from build123d import *

# Parameters (mm, degrees)
SKETCH1_W               = 500
SKETCH1_H               = 200
BOSS_EXTRUDE1_DEPTH     = 100
SKETCH2_R               = 40
BOSS_EXTRUDE2_DEPTH     = 10
SKETCH5_R               = 1.5
CUT_EXTRUDE3_DEPTH      = 20
CIRPATTERN2_COUNT       = 3
MIRROR4_COPY_1_SKETCH_R = 1.5
MIRROR4_COPY_1_DEPTH    = 20
MIRROR4_COPY_2_SKETCH_R = 1.5
MIRROR4_COPY_2_DEPTH    = 20
MIRROR5_COPY_1_SKETCH_R = 1.5
MIRROR5_COPY_1_DEPTH    = 20
MIRROR5_COPY_2_SKETCH_R = 1.5
MIRROR5_COPY_2_DEPTH    = 20
MIRROR5_COPY_3_SKETCH_R = 40
MIRROR5_COPY_3_DEPTH    = 10
MIRROR5_COPY_4_SKETCH_R = 1.5
MIRROR5_COPY_4_DEPTH    = 20
MIRROR5_COPY_5_SKETCH_R = 1.5
MIRROR5_COPY_5_DEPTH    = 20
MIRROR5_COPY_6_SKETCH_R = 1.5
MIRROR5_COPY_6_DEPTH    = 20


with BuildPart() as part:
    # Sketch1 → Boss-Extrude1 (new body)
    with BuildSketch(Plane(origin=(0, 0, 0), x_dir=(1, 0, 0), z_dir=(0, 1, 0))):
        Rectangle(SKETCH1_W, SKETCH1_H)
    extrude(amount=BOSS_EXTRUDE1_DEPTH)

    # Sketch2 → Boss-Extrude2 (add)
    with BuildSketch(Plane.XY.offset(100)):
        with Locations(Location((-170, 50, 0), (0, 0, 180))):
            Circle(SKETCH2_R)
    boss_extrude2 = extrude(amount=BOSS_EXTRUDE2_DEPTH)

    # Sketch5 → Cut-Extrude3 (cut)
    with BuildSketch(Plane.XY.offset(110)):
        with Locations((-170, 86)):
            Circle(SKETCH5_R)
    cut_extrude3 = extrude(amount=-CUT_EXTRUDE3_DEPTH, mode=Mode.SUBTRACT)

    # CirPattern2: Cut-Extrude3 ×3 about axis
    cirpattern2_axis = Axis((-170, 50, 0), (0, 0, 1))
    for i in range(1, CIRPATTERN2_COUNT):
        add(cut_extrude3.rotate(cirpattern2_axis, i * 360 / CIRPATTERN2_COUNT), mode=Mode.SUBTRACT)

    # Mirror4: Boss-Extrude2, Cut-Extrude3 across plane
    add(boss_extrude2.mirror(Plane(origin=(0, 0, 0), x_dir=(0, 0, 1), z_dir=(1, 0, 0))))
    add(cut_extrude3.mirror(Plane(origin=(0, 0, 0), x_dir=(0, 0, 1), z_dir=(1, 0, 0))), mode=Mode.SUBTRACT)

    # Mirror4 copy 1 sketch → Mirror4 copy 1 (cut)
    with BuildSketch(Plane(origin=(211.698729811, 222.224318643, 110), x_dir=(0.4999999999999998, 0.8660254037844387, 0), z_dir=(0, 0, 1))):
        with Locations((-170, -86)):
            Circle(MIRROR4_COPY_1_SKETCH_R)
    extrude(amount=-MIRROR4_COPY_1_DEPTH, mode=Mode.SUBTRACT)

    # Mirror4 copy 2 sketch → Mirror4 copy 2 (cut)
    with BuildSketch(Plane(origin=(298.301270189, -72.224318643, 110), x_dir=(0.5000000000000004, -0.8660254037844384, 0), z_dir=(0, 0, 1))):
        with Locations((-170, -86)):
            Circle(MIRROR4_COPY_2_SKETCH_R)
    extrude(amount=-MIRROR4_COPY_2_DEPTH, mode=Mode.SUBTRACT)

    # Mirror5: Boss-Extrude2, Cut-Extrude3 across plane
    add(boss_extrude2.mirror(Plane.XY))
    add(cut_extrude3.mirror(Plane.XY), mode=Mode.SUBTRACT)

    # Mirror5 copy 1 sketch → Mirror5 copy 1 (cut)
    with BuildSketch(Plane(origin=(-211.698729811, 222.224318643, -110), x_dir=(-0.4999999999999998, 0.8660254037844387, 0), z_dir=(0, 0, -1))):
        with Locations((-170, -86)):
            Circle(MIRROR5_COPY_1_SKETCH_R)
    extrude(amount=-MIRROR5_COPY_1_DEPTH, mode=Mode.SUBTRACT)

    # Mirror5 copy 2 sketch → Mirror5 copy 2 (cut)
    with BuildSketch(Plane(origin=(-298.301270189, -72.224318643, -110), x_dir=(-0.5000000000000004, -0.8660254037844384, 0), z_dir=(0, 0, -1))):
        with Locations((-170, -86)):
            Circle(MIRROR5_COPY_2_SKETCH_R)
    extrude(amount=-MIRROR5_COPY_2_DEPTH, mode=Mode.SUBTRACT)

    # Mirror5 copy 3 sketch → Mirror5 copy 3 (add)
    with BuildSketch(Plane(origin=(0, 0, -100), x_dir=(-1, 0, 0), z_dir=(0, 0, -1))):
        with Locations(Location((-170, 50, 0), (0, 0, 180))):
            Circle(MIRROR5_COPY_3_SKETCH_R)
    extrude(amount=MIRROR5_COPY_3_DEPTH)

    # Mirror5 copy 4 sketch → Mirror5 copy 4 (cut)
    with BuildSketch(Plane(origin=(0, 0, -110), x_dir=(-1, 0, 0), z_dir=(0, 0, -1))):
        with Locations((-170, 86)):
            Circle(MIRROR5_COPY_4_SKETCH_R)
    extrude(amount=-MIRROR5_COPY_4_DEPTH, mode=Mode.SUBTRACT)

    # Mirror5 copy 5 sketch → Mirror5 copy 5 (cut)
    with BuildSketch(Plane(origin=(211.698729811, 222.224318643, -110), x_dir=(0.4999999999999998, 0.8660254037844387, 0), z_dir=(0, 0, -1))):
        with Locations((-170, 86)):
            Circle(MIRROR5_COPY_5_SKETCH_R)
    extrude(amount=-MIRROR5_COPY_5_DEPTH, mode=Mode.SUBTRACT)

    # Mirror5 copy 6 sketch → Mirror5 copy 6 (cut)
    with BuildSketch(Plane(origin=(298.301270189, -72.224318643, -110), x_dir=(0.5000000000000004, -0.8660254037844384, 0), z_dir=(0, 0, -1))):
        with Locations((-170, 86)):
            Circle(MIRROR5_COPY_6_SKETCH_R)
    extrude(amount=-MIRROR5_COPY_6_DEPTH, mode=Mode.SUBTRACT)


solid = part.part
Model file for the job. Use its own axes, mm. A direction names the side the tool comes from. Coordinates: 2 decimals unless noted, no trailing zeros. Loops run counter-clockwise (first coordinate to the right, second up) from the corner with the lowest first, then second, coordinate; pieces in that order, holes last. Notation, with made-up numbers: (6, -23.5) -> (23, -23.5) arc R14 cw to (23, -16.5) -> close; hole circle Ø8 at (61, 83). An arc over 180 degrees is marked (long way). Use one line per item in the form item = value. Start each with the question number.
(1) Tool access for faces 1 (the flat face through (-169, 49, -110)), 2 (the cylindrical face through (130.04, 48.24, 104.93)), 3 (the cylindrical face through (130.04, 48.24, -104.93)): list every direction of +Z, -Z, +X, -X, +Y, -Y with a clear straight run to the whole face (end or side of a thin tool).
(2) Flat gauge pins, fed straight in: pin 1 (2 mm diameter, centred on x = 124.5, z = 76, fed in from -Y); pin 2 (12 mm diameter, centred on x = 111, y = 55, fed in from +Z); pin 3 (1.8 mm diameter, centred on x = 138.82, y = 32, fed in from +Z). Where does each tip first touch, or does it go through?
(3) Pull direction X, two halves, no side cores. Call faces 4 (the flat face through (250, 49, 1)), 5 (the flat face through (169, 49, 110)), 6 (the cylindrical face through (-130.04, 48.24, -104.93)), 7 (the cylindrical face through (-130.04, 48.24, 104.93)): pulls with the +X half, pulls with the -X half, needs draft (parallel to the pull), parting line crosses it, or undercut.
(4) Probe probe 1 along Y at (x, z) = (170, 99); probe 2 along Y at (x, z) = (170, -105.25); probe 3 along Z at (x, y) = (54.5, 37). List the from-to ranges inside material, lowest first. Write a range as from..to.
(5) Cut at B-B on x = 111. Give the cut face in (y, z).
(6) Cut at A-A on y = 50. Give the cut face in (x, z).
Values:
q1.face_1 = -Z, +X, -X, +Y, -Y
q1.face_2 = +Z
q1.face_3 = -Z
q2.pin_1 = 0
q2.pin_2 = 100
q2.pin_3 = 90
q3.face_4 = pulls with the +X half
q3.face_5 = needs draft
q3.face_6 = undercut
q3.face_7 = undercut
q4.probe_1 = 0..84.5, 87.5..100
q4.probe_2 = 10..84.5, 87.5..90
q4.probe_3 = -100..100
q5.outline = (0, -100) -> (100, -100) -> (100, 100) -> (0, 100) -> close
q6.outline = (-250, -100) -> (-210, -100) -> (-210, -110) -> (-130, -110) -> (-130, -100) -> (130, -100) -> (130, -110) -> (210, -110) -> (210, -100) -> (250, -100) -> (250, 100) -> (210, 100) -> (210, 110) -> (130, 110) -> (130, 100) -> (-130, 100) -> (-130, 110) -> (-210, 110) -> (-210, 100) -> (-250, 100) -> close
